Geometry check sheet. Reference: the model listing, model coordinates, mm. A direction names the side the tool comes from. Coordinates: 2 decimals unless noted, no trailing zeros. Loops run counter-clockwise (first coordinate to the right, second up) from the corner with the lowest first, then second, coordinate; pieces in that order, holes last. Notation, with made-up numbers: (10, 32) -> (24, 32) arc R23 cw to (24, 46) -> close; hole circle Ø5 at (33.5, 76). An arc over 180 degrees is marked (long way). Answer as a JSON object with one key per item and string values.
from build123d import *

# Parameters (mm, degrees)
SKETCH1_R           = 15
BOSS_EXTRUDE1_DEPTH = 10
SKETCH2_W           = 10
SKETCH2_H           = 60
BOSS_EXTRUDE2_DEPTH = 60


with BuildPart() as part:
    # Sketch1 → Boss-Extrude1 (new body)
    with BuildSketch(Plane(origin=(0, 0, 0), x_dir=(1, 0, 0), z_dir=(0, 1, 0))):
        with BuildLine():
            Line((0, 30), (0, -30))
            Line((0, -30), (150, -30))
            ThreePointArc((150, -30), (180, 0), (150, 30))
            Line((150, 30), (0, 30))
        make_face()
        with Locations((150, 0)):
            Circle(SKETCH1_R, mode=Mode.SUBTRACT)
    boss_extrude1 = extrude(amount=BOSS_EXTRUDE1_DEPTH)

    # Sketch2 → Boss-Extrude2 (add)
    with BuildSketch(Plane(origin=(0, 10, 0), x_dir=(1, 0, 0), z_dir=(0, 1, 0))):
        with Locations((5, 0)):
            Rectangle(SKETCH2_W, SKETCH2_H)
    extrude(amount=BOSS_EXTRUDE2_DEPTH)

    # Mirror2: Boss-Extrude1 across plane
    add(boss_extrude1.mirror(Plane.ZX.offset(35)))


solid = part.part
1. Tool access check on faces 5 (the face through (94, 60, 0)), 6 (the face through (179.993, 65.07, 0.66)). Record the directions out of +Z, -Z, +X, -X, +Y, -Y that give a thin tool (end or side, any length) a straight path to the whole face; none if there is none.
Evaluation:
{"face 5": "+Z, -Z, +X", "face 6": "+X, +Y, -Y"}
2. Section check D-D, the plane y = 7.5. Record the boundary of the cut face in (x, z), then the cut area to 3 significant figures.
Evaluation:
{"outline": "(0, -30) -> (150, -30) arc R30 ccw to (150, 30) -> (0, 30) -> close; hole circle Ø30 at (150, 0)", "area": "9,710 mm^2"}
3. Section check A-A, the plane x = 78. Record the boundary of the cut face in (y, z), then the cut area to 3 significant figures.
Evaluation:
{"outline": "(0, -30) -> (10, -30) -> (10, 30) -> (0, 30) -> close; (60, -30) -> (70, -30) -> (70, 30) -> (60, 30) -> close", "area": "1,200 mm^2"}
4. Depth check by flat-ended pin: P1, Ø5, axis at y = 41.5, z = -23.5, coming from the +X side; P2, Ø12, axis at y = 11, z = -5, coming from the +X side. Enter the tip coordinate at first touch or a pass-through.
Evaluation:
{"P1": "stops at x = 10", "P2": "stops at x = 180"}
5. Section check B-B, the plane z = 0. Record the boundary of the cut face in (x, y).
Evaluation:
{"outline": "(0, 0) -> (135, 0) -> (135, 10) -> (10, 10) -> (10, 60) -> (135, 60) -> (135, 70) -> (0, 70) -> close; (165, 0) -> (180, 0) -> (180, 10) -> (165, 10) -> close; (165, 60) -> (180, 60) -> (180, 70) -> (165, 70) -> close"}
6. Thickness scan on probe 1 along Z at (x, y) = (150, 4); probe 2 along X at (y, z) = (2.75, 0); probe 3 along Y at (x, z) = (171.5, 4). Record the ranges inside material, lowest first. Write a range as from..to.
Evaluation:
{"probe 1": "z = -30..-15, 15..30", "probe 2": "x = 0..135, 165..180", "probe 3": "y = 0..10, 60..70"}
7. Mould release check, pull along Z, two halves, no side actions. Record for faces 1 (the face through (0, 35, 0)), 2 (the face through (135.015, 4.93, -0.66)), 3 (the face through (135.015, 65.07, -0.66)), 4 (the face through (179.993, 4.93, 0.66)): released by +Z, released by -Z, zero draft, split by the parting line, or undercut.
Evaluation:
{"face 1": "zero draft", "face 2": "undercut", "face 3": "undercut", "face 4": "split by the parting line"}
8. Section check C-C, the plane x = 144.5. Record the boundary of the cut face in (y, z), then the cut area to 3 significant figures.
Evaluation:
{"outline": "(0, -30) -> (10, -30) -> (10, -13.96) -> (0, -13.96) -> close; (0, 13.96) -> (10, 13.96) -> (10, 30) -> (0, 30) -> close; (60, -30) -> (70, -30) -> (70, -13.96) -> (60, -13.96) -> close; (60, 13.96) -> (70, 13.96) -> (70, 30) -> (60, 30) -> close", "area": "642 mm^2"}
